Study the drawing (mm; zero at the part's minimum x, y, z) and answer. Coordinates: 2 decimals unless noted, no trailing zeros. Order: outer loops, then holes, each group sorted by start corner. A loop starts at its lowest first (then second) coordinate and runs counter-clockwise, first axis right, second up. Notation, with made-up numbers: M 63,-29 L 71,-29 A30 ccw 71,10 Z; hole C 58,19.5 d10. An arc over 180 degrees is marked long. One line per item, written item: value. Start each with the question number.
Q1. Straight lines are drawn through the part: line 1 along Y through (x, z) = (95, 1.6); line 2 along X through (y, z) = (5.25, 2.7); line 3 along X through (y, z) = (13, 2). For each, find the intervals that lie inside material, in ascending order. Write a range as [from, to].
Q2. The part is cut by section C-C on y = 7.75. Give the vertices of the cut face in (x, z), then the cut area to 3 significant figures.
Q3. The part is cut by section A-A on x = 95. Give the vertices of the cut face in (y, z).
Q4. The part is cut by section B-B on z = 2.05. Give the number of separate pieces and of enclosed holes in the cut face, then the cut area to 3 significant figures.
Q5. This flat-tipped pin is pushed along its axis until it touches: pin 1 Ø9.5 at (x, y) = (95, 10) entering from -Z. Where does it stop, or does it pass through?
Q6. The part is cut by section D-D on y = 18. Give the vertices of the cut face in (x, z), then the cut area to 3 significant figures.
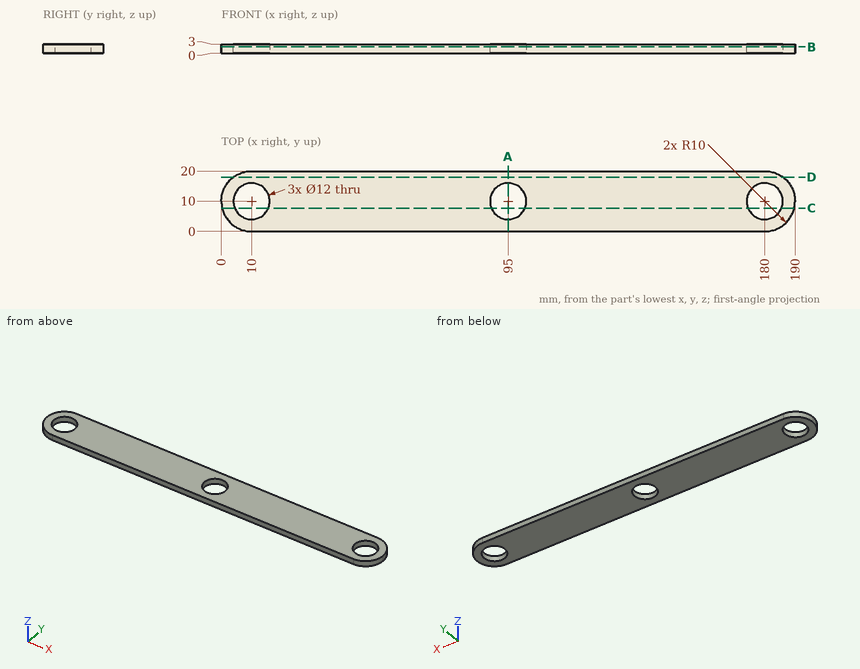
Output:
1. line 1: y = [0, 4], [16, 20]
1. line 2: x = [1.2, 6.33], [13.67, 91.33], [98.67, 176.33], [183.67, 188.8]
1. line 3: x = [0.46, 4.8], [15.2, 89.8], [100.2, 174.8], [185.2, 189.54]
2. outline: M 0.26,0 L 4.44,0 L 4.44,3 L 0.26,3 Z; M 15.56,0 L 89.44,0 L 89.44,3 L 15.56,3 Z; M 100.56,0 L 174.44,0 L 174.44,3 L 100.56,3 Z; M 185.56,0 L 189.74,0 L 189.74,3 L 185.56,3 Z
2. area: 468 mm^2
3. outline: M 0,0 L 4,0 L 4,3 L 0,3 Z; M 16,0 L 20,0 L 20,3 L 16,3 Z
4. separate pieces: 1
4. enclosed holes: 3
4. area: 3,370 mm^2
5. pin 1: passes through
6. outline: M 4,0 L 186,0 L 186,3 L 4,3 Z
6. area: 546 mm^2
